Can you work these out from the model? Positions are in its coordinate system, mm. Round coordinates to 2 decimals unless told otherwise and drop trailing zeros. Loops run counter-clockwise (first coordinate to the right, second up) from the corner with the lowest first, then second, coordinate; pieces in that order, holes last.
from build123d import *

# Parameters (mm, degrees)
SKETCH1_R          = 375.92
SKETCH1_R_2        = 342.9
EXTRUDE1_DEPTH     = 3.175
SKETCH2_R          = 3.556
CUT_EXTRUDE1_DEPTH = 3.175
CIRPATTERN1_COUNT  = 20
CUT_EXTRUDE3_DEPTH = 3.175
CIRPATTERN2_COUNT  = 10


with BuildPart() as part:
    # Sketch1 → Extrude1 (new body)
    with BuildSketch(Plane.XY):
        Circle(SKETCH1_R)
        Circle(SKETCH1_R_2, mode=Mode.SUBTRACT)
    extrude(amount=EXTRUDE1_DEPTH)

    # Sketch2 → Cut-Extrude1 (cut)
    with BuildSketch(Plane.XY.offset(3.175)):
        with Locations((0, -358.775)):
            Circle(SKETCH2_R)
    cut_extrude1 = extrude(amount=-CUT_EXTRUDE1_DEPTH, mode=Mode.SUBTRACT)

    # CirPattern1: Cut-Extrude1 ×20 about axis
    cirpattern1_axis = Axis((0, 0, 0), (0, 0, 1))
    for i in range(1, CIRPATTERN1_COUNT):
        add(cut_extrude1.rotate(cirpattern1_axis, i * 360 / CIRPATTERN1_COUNT), mode=Mode.SUBTRACT)

    # Sketch3 → Cut-Extrude3 (cut)
    with BuildSketch(Plane.XY.offset(3.175)):
        Polygon((168.294733652, -336.143911182), (61.426903046, -370.867337443), (-61.427134053, -370.867299181), (-80.587451942, -486.54802329), (220.789134468, -440.993735193), align=None)
    cut_extrude3 = extrude(amount=-CUT_EXTRUDE3_DEPTH, mode=Mode.SUBTRACT)

    # CirPattern2: Cut-Extrude3 ×10 about axis
    cirpattern2_axis = Axis((0, 0, 0), (0, 0, 1))
    for i in range(1, CIRPATTERN2_COUNT):
        add(cut_extrude3.rotate(cirpattern2_axis, i * 360 / CIRPATTERN2_COUNT), mode=Mode.SUBTRACT)


solid = part.part
(1) If we mould it in two halves opening along Y, with no side actions, what happens to faces 1 (the cylindrical face through (184.341, 289.135, 1.565)), 2 (the flat face through (-301.172, 217.842, 1.61)), 3 (the flat face through (-217.295, -300.543, 1.61))? For each: released by +Y, released by -Y, zero draft, split by the parting line, or undercut.
Worked answers:
face 1: undercut
face 2: released by +Y
face 3: released by -Y
(2) If we section it at C-C, the plane z = 2.5: State how many separate pieces and enclosed holes the cut face has, then the cut area to 3 significant figures.
Worked answers:
separate pieces: 1
enclosed holes: 21
area: 66,500 mm2
(3) If I drill on line 1 (X direction, y = 5, z = 1.1); line 2 (Y direction, x = 0, z = 2.4); line 3 (Y direction, x = -290.5, z = 2.9), over which ranges is the centre line in solid material (lowest first)?
Worked answers:
line 1: x = -371.7 to -342.86, 342.86 to 371.7
line 2: y = -370.87 to -362.33, -355.22 to -342.9, 342.9 to 355.22, 362.33 to 370.87
line 3: y = -232.53 to -214.43, -207.34 to -182.18, 182.18 to 207.34, 214.43 to 232.53
(4) Will this pin go through, and if not, where does the flat tip stop? P1, Ø1, axis at x = 166, z = 0.5, coming from the -Y side.
Worked answers:
P1: stops at y = -337.05
(5) If we section it at B-B, the plane y = -226: List the corners of the cut face in (x, z) for me (3 decimals).
Worked answers:
outline: (-295.245, 0) - (-257.884, 0) - (-257.884, 3.175) - (-295.245, 3.175) - close; (257.884, 0) - (295.245, 0) - (295.245, 3.175) - (257.884, 3.175) - close
(6) If we section it at A-A, the plane x = -40: List the corners of the cut face in (y, z) for me (3 decimals).
Worked answers:
outline: (-370.867, 0) - (-340.559, 0) - (-340.559, 3.175) - (-370.867, 3.175) - close; (340.559, 0) - (370.867, 0) - (370.867, 3.175) - (340.559, 3.175) - close
